Verification items for this drawing (mm, ordinates from the low corner). A direction names the side the tool comes from. Round coordinates to 2 decimals unless told otherwise and drop trailing zeros. Write each loop counter-clockwise with the first axis right and the second up, starting at its lowest first coordinate (ties: lowest second). Pieces come first, ordered by that corner, then holes. Notation, with made-up numbers: (38.25, -1.5) -> (51.25, -1.5) arc R20 cw to (51.25, 21.5) -> close; hole circle Ø8 at (-22, 1). An arc over 180 degrees is marked (long way). One line per question, with ' | ' between items.
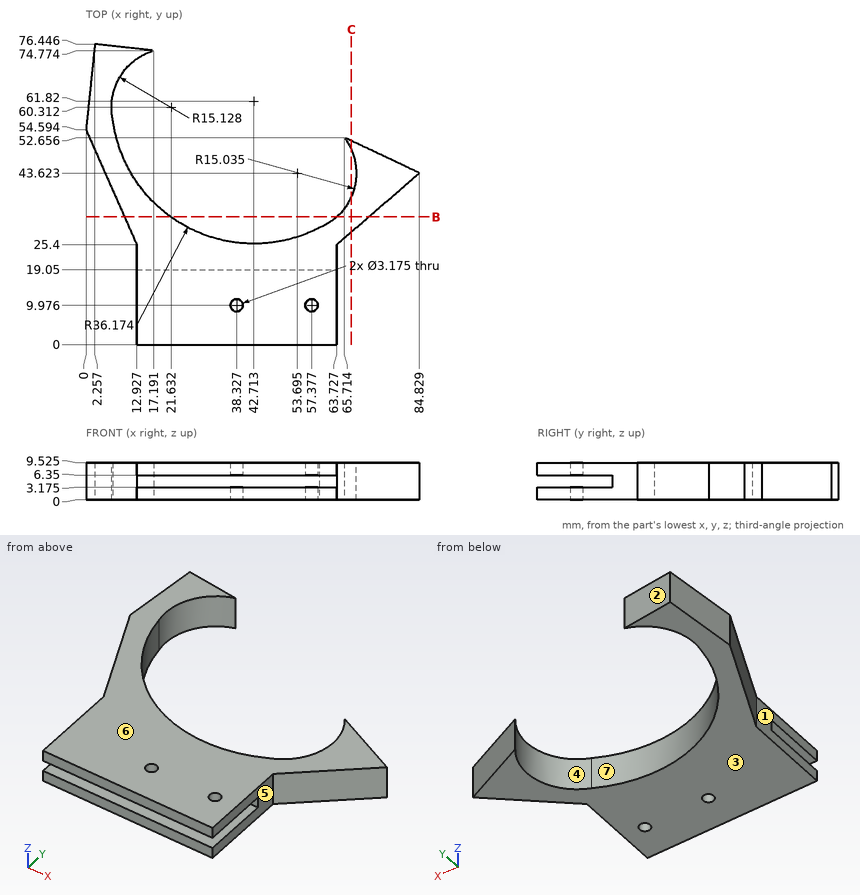
(1) Draft check along X on the marked faces 1, 2, 3 and 4. Enter one of: +X half, -X half, draft (parallel to the pull), parting line (faces both ways), or undercut.
Resolved:
face 1: -X half | face 2: +X half | face 3: draft | face 4: undercut
(2) Sectioned sample at C-C on x = 67.5. Record the cut outline in (y, z) (1 decimal).
Resolved:
outline: (28.7, 0) -> (37.7, 0) -> (37.7, 9.5) -> (28.7, 9.5) -> close; (49.6, 0) -> (51.8, 0) -> (51.8, 9.5) -> (49.6, 9.5) -> close
(3) Material ranges on line 1 (X direction, y = 13.5, z = 9); line 2 (X direction, y = 46, z = 2.5) (1 decimal); line 3 (X direction, y = 35, z = 9) (1 decimal), recorded low to high.
Resolved:
line 1: x = 12.93 to 63.73 | line 2: x = 3.8 to 10.2, 68.5 to 79.8 | line 3: x = 8.7 to 18.4, 66 to 74.8
(4) Access from +Z, -Z, +X, -X, +Y, -Y to the whole of each face (thin tool, end or side, straight path). Record for the marked faces 5, 6 and 7.
Resolved:
face 5: +Z, -Z, +X, -Y | face 6: +Z, +X, -X, +Y, -Y | face 7: +Z, -Z
(5) Sectioned sample at B-B on y = 32.5. Record the cut outline in (x, z) (1 decimal).
Resolved:
outline: (9.8, 0) -> (21.5, 0) -> (21.5, 9.5) -> (9.8, 9.5) -> close; (63.8, 0) -> (71.9, 0) -> (71.9, 9.5) -> (63.8, 9.5) -> close
(6) Go/stop test with flat-tipped pins: pin 1 (1.9 mm diameter, centred on x = 38.33, y = 9.98, fed in from -Z); pin 2 (5 mm diameter, centred on y = 53.5, z = 4.5, fed in from +X) (1 decimal); pin 3 (5 mm diameter, centred on y = 68.5, z = 7.5, fed in from +X) (1 decimal); pin 4 (21 mm diameter, centred on x = 39.5, y = 5, fed in from -Z). Record where each tip stops, or that it passes through.
Resolved:
pin 1: passes through | pin 2: stops at x = 69.2 | pin 3: stops at x = 10.9 | pin 4: stops at z = 0
